Design review of the part shown in the three views and the two pictorial views. Dimensions are in mm from the part's minimum x, y and z. A direction names the side the tool comes from. Round coordinates to 2 decimals unless told otherwise and drop trailing zeros. Order: outer loops, then holes, each group sorted by start corner. A loop starts at its lowest first (then second) coordinate and runs counter-clockwise, first axis right, second up. Notation, with made-up numbers: M 9.25,25 L 53.25,25 A35 ccw 53.25,58 Z; hole C -24.75,46 d9. An arc over 180 degrees is marked long. Write item = value, one per line. Start each with the question number.
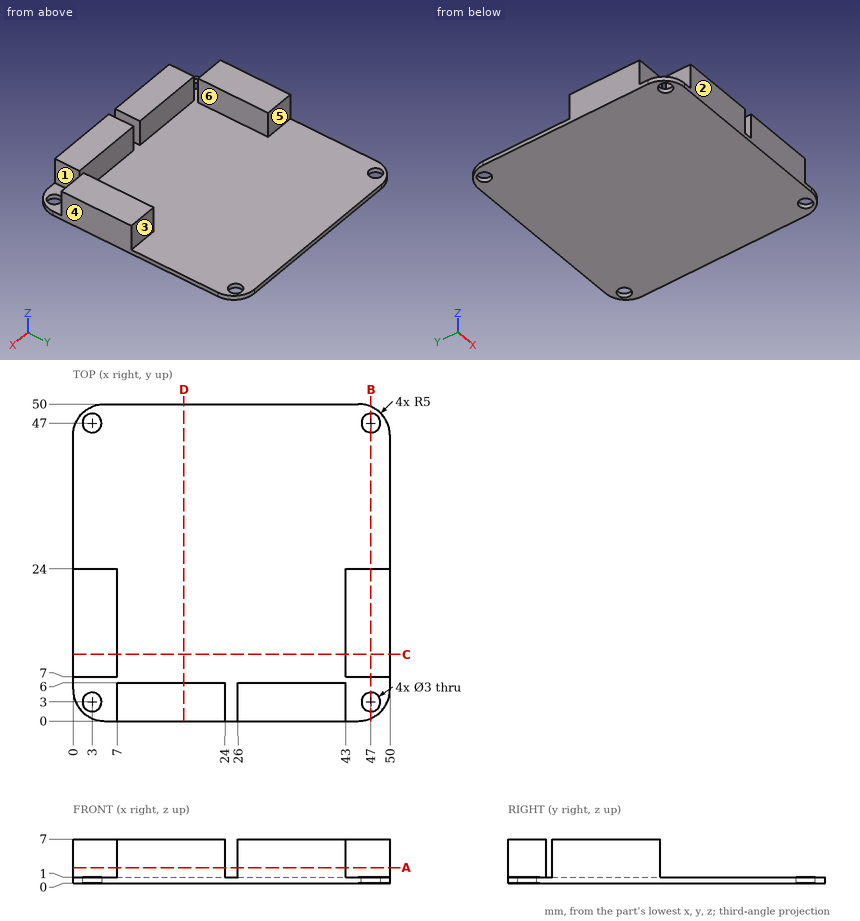
(1) For the marked faces 1, 2 and 3, list the 3-axis set-ups (+Z, -Z, +X, -X, +Y, -Y) from which the entire face can be reached by the end or side of a thin tool; tool diameter is ignored.
(2) We need section B-B, the plane x = 47. Write out the cut boundary in (y, z), then the cut area to 3 significant figures.
(3) Insertion check: pin 1 (4 mm diameter, centred on x = 17, z = 3, fed in from -Y); pin 2 (4 mm diameter, centred on x = 47, y = 47, fed in from +Z); pin 3 (3 mm diameter, centred on x = 2.5, z = 3.5, fed in from +Y); pin 4 (3 mm diameter, centred on x = 47.5, z = 4, fed in from -Y). Each pin has a flat end and moves straight along its axis. Give the tip position at first contact, or say it passes through.
(4) Draft analysis for pull direction X (two halves, no side actions). For the marked faces 4, 5 and 6, state which applies: released by +X, released by -X, zero draft, split by the parting line, or undercut.
(5) For line 1 along X through (y, z) = (10, 5.75); line 2 along Y through (x, z) = (47, 0.6); line 3 along Z through (x, y) = (17.5, 11.5), list the stretches that pass through material, from the lowest coordinate up.
(6) We need section D-D, the plane x = 17.5. Write out the cut boundary in (y, z), then the cut area to 3 significant figures.
(7) We need section A-A, the plane z = 2.5. Write out the cut boundary in (x, y), then the cut area to 3 significant figures.
(8) We need section C-C, the plane y = 10.5. Write out the cut boundary in (x, z), then the cut area to 3 significant figures.
Values:
q1.face_1 = +Z, +X, -Y
q1.face_2 = +Z, -Z, +X, -X, -Y
q1.face_3 = +Z, +X, -X, +Y
q2.outline = M 0.42,0 L 1.5,0 L 1.5,1 L 0.42,1 Z; M 4.5,0 L 45.5,0 L 45.5,1 L 24,1 L 24,7 L 7,7 L 7,1 L 4.5,1 Z; M 48.5,0 L 49.58,0 L 49.58,1 L 48.5,1 Z
q2.area = 145 mm²
q3.pin_1 = 0
q3.pin_2 = 1
q3.pin_3 = 24
q3.pin_4 = 7
q4.face_4 = released by +X
q4.face_5 = zero draft
q4.face_6 = undercut
q5.line_1 = 0 to 7, 43 to 50
q5.line_2 = 0.42 to 1.5, 4.5 to 45.5, 48.5 to 49.58
q5.line_3 = 0 to 1
q6.outline = M 0,0 L 50,0 L 50,1 L 6,1 L 6,7 L 0,7 Z
q6.area = 86.0 mm²
q7.outline = M 0,7 L 7,7 L 7,24 L 0,24 Z; M 7,0 L 24,0 L 24,6 L 7,6 Z; M 26,0 L 43,0 L 43,6 L 26,6 Z; M 43,7 L 50,7 L 50,24 L 43,24 Z
q7.area = 442 mm²
q8.outline = M 0,0 L 50,0 L 50,7 L 43,7 L 43,1 L 7,1 L 7,7 L 0,7 Z
q8.area = 134 mm²
